Answer from the drawing. Dimensions are ordinates in mm from the lowest x, y and z of the part. A direction names the side the tool comes from. Coordinates: 2 decimals unless noted, no trailing zeros. Write each loop counter-clockwise with the first axis right and the second up, starting at its lowest first coordinate (ties: lowest second). Pieces come first, ordered by that corner, then holes.
(1) The mould has two halves that part along X. Classify the marked faces 3, 4 and 5: +X half, -X half, draft (parallel to the pull), parting line (faces both ways), or undercut.
(2) Which of the six approach directions +Z, -Z, +X, -X, +Y, -Y give full straight-line access (tool end or side, diameter ignored) to the marked faces 1 and 2?
(3) Section B-B on z = 3 is taken. Write down the section's boundary in (x, y), then the cut area to 4 significant figures.
(4) Find the intervals of material crossed by probe 1 along X at (y, z) = (2.75, 9); probe 2 along X at (y, z) = (0.75, 2.5); probe 3 along Y at (x, z) = (9, 11.75), in increasing order.
(5) Section C-C on x = 58 is taken. Write down the section's boundary in (y, z).
(6) Section A-A on y = 3.75 is taken. Write down the section's boundary in (x, z), then the cut area to 3 significant figures.
(7) Given pin 1 (4 mm diameter, centred on x = 62, z = 5.5, fed in from -Y), flat-ended and moving along its own axis, determine where the tip first touches the part or whether it passes through.
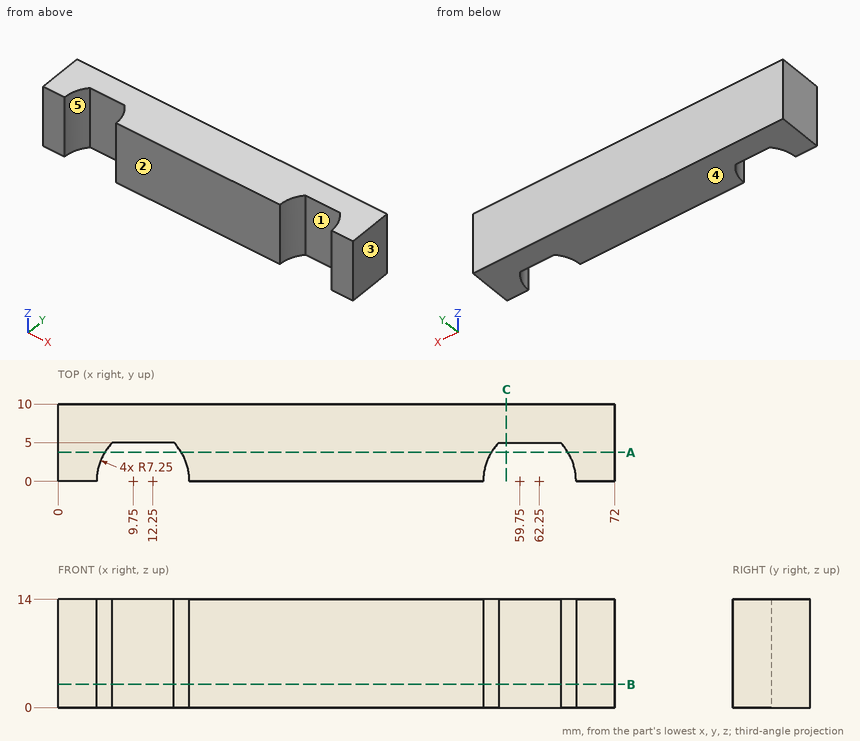
Response:
1. face 3: +X half
1. face 4: draft
1. face 5: undercut
2. face 1: +Z, -Z, -Y
2. face 2: +Z, -Z, +X, -X, -Y
3. outline: (0, 0) - (5, 0) arc R7.25 cw to (7, 5) - (15, 5) arc R7.25 cw to (17, 0) - (55, 0) arc R7.25 cw to (57, 5) - (65, 5) arc R7.25 cw to (67, 0) - (72, 0) - (72, 10) - (0, 10) - close
3. area: 612.5 mm2
4. probe 1: x = 0 to 5.54, 16.46 to 55.54, 66.46 to 72
4. probe 2: x = 0 to 5.04, 16.96 to 55.04, 66.96 to 72
4. probe 3: y = 5 to 10
5. outline: (5, 0) - (10, 0) - (10, 14) - (5, 14) - close
6. outline: (0, 0) - (6.05, 0) - (6.05, 14) - (0, 14) - close; (15.95, 0) - (56.05, 0) - (56.05, 14) - (15.95, 14) - close; (65.95, 0) - (72, 0) - (72, 14) - (65.95, 14) - close
6. area: 731 mm2
7. pin 1: stops at y = 5
